```python
from build123d import *

# Parameters (mm, degrees)
F0_W     = 449.5038
F0_H     = 127
F0_R     = 44.5643
F1_DEPTH = 50.8
F2_DEPTH = 50.8


with BuildPart() as f1:
    # F0 (on Top) → F1 (new body)
    with BuildSketch(Plane.XY):
        with Locations((23.634577, -3.505918)):
            Rectangle(F0_W, F0_H)
        with Locations((23.634577, -3.505918)):
            Circle(F0_R, mode=Mode.SUBTRACT)
    extrude(amount=F1_DEPTH)

    # F0 (on Top) → F2 (join)
    with BuildSketch(Plane.XY):
        with Locations((23.634577, -3.505918)):
            Rectangle(F0_W, F0_H)
        with Locations((23.634577, -3.505918)):
            Circle(F0_R, mode=Mode.SUBTRACT)
    extrude(amount=F2_DEPTH)


solid = f1.part
```
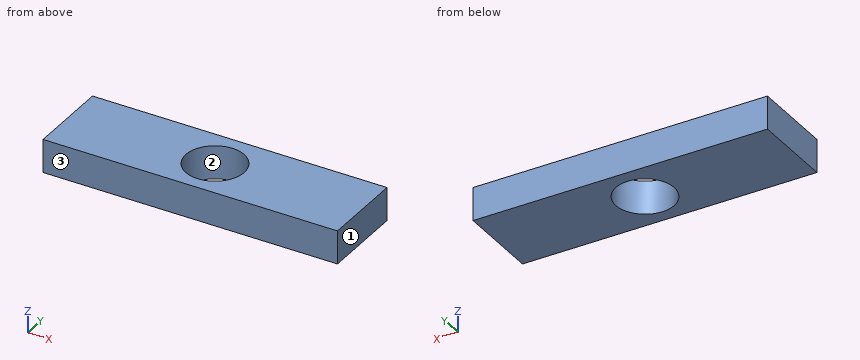
Design review of the part built by this model. Coordinates are the model's own, in mm. Face numbers are marked on the shaded views. Coordinates: 2 decimals unless noted, no trailing zeros. Write each loop counter-clockwise with the first axis right and the second up, starting at its lowest first coordinate (ties: lowest second). Pieces come first, ordered by that corner, then holes.
1) Add section B-B (x = 28). Write out the cut boundary in (y, z), plus the area to 3 significant figures.
2) To check wall thickness, follow L1, parallel to X at y = -5.5, z = 26; L2, parallel to X at y = 14, z = 6; L3, parallel to Y at x = 20.5, z = 46. State the ranges of each line that lie inside material, in increasing order.
3) Add section A-A (y = 13). Write out the cut boundary in (x, z).
4) Add section C-C (z = 36.5). Write out the cut boundary in (x, y), plus the area to 3 significant figures.
5) Mouldability with a two-part tool opening along Y and no side actions: class the marked faces 1, 2 and 3 as +Y half, -Y half, draft (parallel to the pull), parting line (faces both ways), or undercut.
6) Insertion check: pin 1 (1 mm diameter, centred on x = 64, y = 42, fed in from -Z). The pin has a flat end and moves straight along its axis. Give the tip position at first contact, or say it passes through.
Check result:
1. outline: (-67.01, 0) - (-47.86, 0) - (-47.86, 50.8) - (-67.01, 50.8) - close; (40.84, 0) - (59.99, 0) - (59.99, 50.8) - (40.84, 50.8) - close
1. area: 1,950 mm2
2. L1: x = -201.12 to -20.89, 68.15 to 248.39
2. L2: x = -201.12 to -17.35, 64.62 to 248.39
2. L3: y = -67.01 to -47.96, 40.95 to 59.99
3. outline: (-201.12, 0) - (-17.76, 0) - (-17.76, 50.8) - (-201.12, 50.8) - close; (65.03, 0) - (248.39, 0) - (248.39, 50.8) - (65.03, 50.8) - close
4. outline: (-201.12, -67.01) - (248.39, -67.01) - (248.39, 59.99) - (-201.12, 59.99) - close; hole circle Ø89.13 at (23.63, -3.51)
4. area: 50,800 mm2
5. face 1: draft
5. face 2: undercut
5. face 3: -Y half
6. pin 1: stops at z = 0
